from build123d import *

# Parameters (mm, degrees)
F1_DEPTH     = 12
F3_DEPTH     = 9
F4_R         = 1.5
F5_DEPTH     = 4
F6_T1_DEPTH  = 12
F6_T3_DEPTH  = 9
F6_T5_DEPTH  = 11.7568277192
F6_T7_DEPTH  = 16.5
F6_T9_DEPTH  = 11.7568277192
F6_T11_DEPTH = 55.4822209965
F6_T13_DEPTH = 27
F6_T15_DEPTH = 42.7993296961
F7_R         = 1


# Not quite as in the source:
# - a fillet or chamfer that OpenCascade refuses, or shapes differently, is made with other operations: its cross-section is extruded or revolved along the edge and cut away or added


with BuildPart() as f1:
    # F0 (on Top) → F1 (new body)
    with BuildSketch(Plane.XY):
        Polygon((-83, 65), (0, 0), (0, 80), (-3, 80), (-3, 65), align=None)
        Polygon((-11.5, 50), (-3, 50), (-3, 29.5), (-11.5, 39.5), align=None, mode=Mode.SUBTRACT)
    extrude(amount=F1_DEPTH)

    # F2 (on face) → F3 (cut)
    with BuildSketch(Plane.XY.offset(12)):
        Polygon((-4, 54), (-4, 61), (-71.4047410676, 61), (-4, 8.2131545856), (-4, 24.5002801184), (-15.5, 38.0296918831), (-15.5, 54), align=None)
    extrude(amount=-F3_DEPTH, mode=Mode.SUBTRACT)

    # F4 (on face) → F5 (cut)
    with BuildSketch(Plane(origin=(0, 65, 0), x_dir=(-1, 0, 0), z_dir=(0, 1, 0))):
        with Locations((50, 7.5)):
            Circle(F4_R)
        with Locations((25, 7.5)):
            Circle(F4_R)
    extrude(amount=-F5_DEPTH, mode=Mode.SUBTRACT)

    # F6: fillet of radius 3 on 12 edges, made by hand

    # F6_s2 → F6_t1 (join)
    with BuildSketch(Plane.XY):
        with BuildLine():
            ThreePointArc((-6, 65), (-3.8786796564, 65.8786796564), (-3, 68))
            Line((-3, 68), (-3, 65))
            Line((-3, 65), (-6, 65))
        make_face()
    extrude(amount=F6_T1_DEPTH)

    # F6_s4 → F6_t3 (join)
    with BuildSketch(Plane.XY.offset(3)):
        with BuildLine():
            ThreePointArc((-4, 57), (-4.8786796564, 54.8786796564), (-7, 54))
            Line((-7, 54), (-4, 54))
            Line((-4, 54), (-4, 57))
        make_face()
        with BuildLine():
            ThreePointArc((-4, 58), (-4.8786796564, 60.1213203436), (-7, 61))
            Line((-7, 61), (-4, 61))
            Line((-4, 61), (-4, 58))
        make_face()
        with BuildLine():
            ThreePointArc((-8.8496919869, 12.0111061416), (-5.6864315702, 11.6758853817), (-4, 14.3730205248))
            Line((-4, 14.3730205248), (-4, 8.2131545856))
            Line((-4, 8.2131545856), (-8.8496919869, 12.0111061416))
        make_face()
        with BuildLine():
            ThreePointArc((-62.7082968683, 61), (-65.544292562, 58.9783294052), (-64.5579888552, 55.6380856168))
            Line((-64.5579888552, 55.6380856168), (-71.4047410676, 61))
            Line((-71.4047410676, 61), (-62.7082968683, 61))
        make_face()
    extrude(amount=F6_T3_DEPTH)

    # F6_s6 → F6_t5 (join)
    with BuildSketch(Plane.XY.offset(0.2431722808)):
        with BuildLine():
            ThreePointArc((-4, 23.3975490307), (-4.1842004812, 24.4325722527), (-4.7141820467, 25.340494291))
            Line((-4.7141820467, 25.340494291), (-4, 24.5002801184))
            Line((-4, 24.5002801184), (-4, 23.3975490307))
        make_face()
    extrude(amount=F6_T5_DEPTH)

    # F6_s8 → F6_t7 (cut)
    with BuildSketch(Plane.XY.offset(3)):
        with BuildLine():
            ThreePointArc((-15.5, 51), (-14.6213203436, 53.1213203436), (-12.5, 54))
            Line((-12.5, 54), (-15.5, 54))
            Line((-15.5, 54), (-15.5, 51))
        make_face()
    extrude(amount=F6_T7_DEPTH, mode=Mode.SUBTRACT)

    # F6_s10 → F6_t9 (cut)
    with BuildSketch(Plane.XY.offset(3)):
        with BuildLine():
            ThreePointArc((-14.7858179533, 37.1894777105), (-15.3157995188, 38.0973997488), (-15.5, 39.1324229708))
            Line((-15.5, 39.1324229708), (-15.5, 38.0296918831))
            Line((-15.5, 38.0296918831), (-14.7858179533, 37.1894777105))
        make_face()
    extrude(amount=F6_T9_DEPTH, mode=Mode.SUBTRACT)

    # F6_s12 → F6_t11 (cut)
    with BuildSketch(Plane.XY.offset(-21.7411104983)):
        with BuildLine():
            ThreePointArc((-76.1532477876, 59.6380856168), (-77.1395514944, 62.9783294052), (-74.3035558007, 65))
            Line((-74.3035558007, 65), (-83, 65))
            Line((-83, 65), (-76.1532477876, 59.6380856168))
        make_face()
    extrude(amount=F6_T11_DEPTH, mode=Mode.SUBTRACT)

    # F6_s14 → F6_t13 (cut)
    with BuildSketch(Plane.XY.offset(-7.5)):
        with BuildLine():
            ThreePointArc((0, 80), (-2.1213203436, 79.1213203436), (-3, 77))
            Line((-3, 77), (-3, 80))
            Line((-3, 80), (0, 80))
        make_face()
        with BuildLine():
            ThreePointArc((0, 77), (-0.8786796564, 79.1213203436), (-3, 80))
            Line((-3, 80), (0, 80))
            Line((0, 80), (0, 77))
        make_face()
    extrude(amount=F6_T13_DEPTH, mode=Mode.SUBTRACT)

    # F6_s16 → F6_t15 (cut)
    with BuildSketch(Plane.XY.offset(-15.399664848)):
        with BuildLine():
            ThreePointArc((-4.8496919869, 3.797951556), (-1.6864315702, 3.4627307961), (0, 6.1598659392))
            Line((0, 6.1598659392), (0, 0))
            Line((0, 0), (-4.8496919869, 3.797951556))
        make_face()
    extrude(amount=F6_T15_DEPTH, mode=Mode.SUBTRACT)

    # F7
    f7_edges = [f1.edges().sort_by_distance(p)[0] for p in [
        (-11.5, 50, 6),
        (-3, 50, 6),
        (-11.5, 39.5, 6),
        (-3, 29.5, 6),
    ]]
    fillet(f7_edges, radius=F7_R)


solid = f1.part
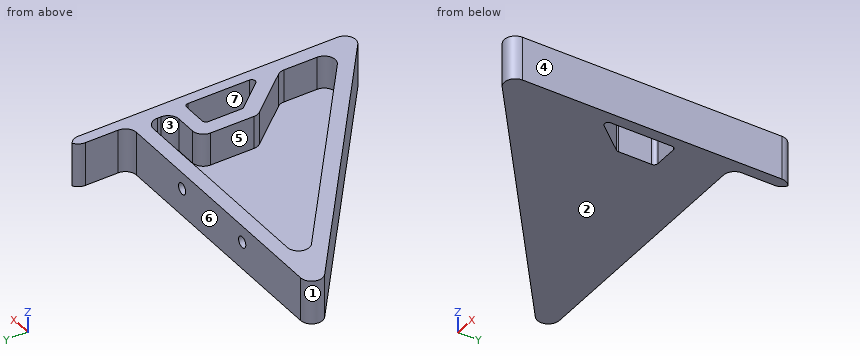
Check sheet for the modelled part. Datum: model origin and axes. Units: mm. Face numbers are marked on the shaded views. A direction names the side the tool comes from. Coordinates: 2 decimals unless noted, no trailing zeros. Write each loop counter-clockwise with the first axis right and the second up, starting at its lowest first coordinate (ties: lowest second). Pieces come first, ordered by that corner, then holes. Notation, with made-up numbers: M 68,-8.5 L 108,-8.5 A23 cw 108,8.5 Z; hole C 65.25,-14 d5. An arc over 180 degrees is marked long. Answer as CSV lines item,"result".
Q1. Set-up check for the marked faces 4, 5, 6 and 7: record each of +Z, -Z, +X, -X, +Y, -Y from which the full face is reachable in a straight line by a thin tool's end or side.
Check result:
face 4,"+Z, -Z, +X, +Y, -Y"
face 5,"+Z"
face 6,"+Z, -Z, -X, +Y"
face 7,"+Z, -Z"
Q2. Cross-section at D-D (x = -46). Record the boundary of the cut face in (y, z), then the cut area to 3 significant figures.
Check result:
outline,"M 36.02,0 L 65,0 L 65,12 L 61,12 L 61,3 L 41.1,3 L 41.1,12 L 36.02,12 Z"
area,"169 mm^2"
Q3. Cross-section at B-B (x = -25.5). Record the boundary of the cut face in (y, z).
Check result:
outline,"M 19.97,0 L 65,0 L 65,6.09 L 61,6.09 L 61,3 L 25.05,3 L 25.05,12 L 19.97,12 Z; M 61,8.91 L 65,8.91 L 65,12 L 61,12 Z"
Q4. Mould release check, pull along Y, two halves, no side actions. Record for the marked faces 1, 2 and 3: released by +Y, released by -Y, zero draft, split by the parting line, or undercut.
Check result:
face 1,"split by the parting line"
face 2,"zero draft"
face 3,"undercut"
Q5. Go/stop test with flat-tipped pins: pin 1 (2 mm diameter, centred on x = -5.5, z = 5, fed in from -Y); pin 2 (1.8 mm diameter, centred on x = -50, z = 7.5, fed in from -Y); pin 3 (3 mm diameter, centred on x = -9.5, z = 6, fed in from +Y). Record where each tip stops, or that it passes through.
Check result:
pin 1,"y = 3.56"
pin 2,"y = 38.45"
pin 3,"y = 65"
Q6. Cross-section at A-A (z = 10.5). Count the separate pieces of the cut face and the enclosed holes in it, then the cut area to 3 significant figures.
Check result:
separate pieces,"1"
enclosed holes,"2"
area,"1,100 mm^2"
Q7. Cross-section at C-C (y = 46.5). Record the boundary of the cut face in (x, z), then the cut area to 3 significant figures.
Check result:
outline,"M -59.38,0 L -11.5,0 L -11.5,12 L -15.5,12 L -15.5,3 L -52.89,3 L -52.89,12 L -59.38,12 Z; M -3,0 L 0,0 L 0,12 L -3,12 Z"
area,"274 mm^2"
Q8. Material ranges on probe 1 along Z at (x, y) = (-25, 62); probe 2 along X at (y, z) = (42, 10.25); probe 3 along X at (y, z) = (17, 7), recorded low to high. Write a range as from..to.
Check result:
probe 1,"0..6, 9..12"
probe 2,"-53.63..-47.14, -15.5..-11.5, -3..0"
probe 3,"-21.71..-15.22, -4..0"
